```python
from build123d import *

# Parameters (mm, degrees)
F0_R     = 1.75
F0_R_2   = 1
F1_DEPTH = 5.6
F3_W     = 0.9
F3_H     = 5.5
F4_DEPTH = 5.95
F5_R     = 3.5
F5_R_2   = 1.75
F6_DEPTH = 4.2
F7_R     = 2.5
F8_DEPTH = 8


with BuildPart() as f1:
    # F0 (on Front) → F1 (new body)
    with BuildSketch(Plane.XZ):
        with BuildLine():
            Line((-26.9, -2), (-26.9, 0))
            ThreePointArc((-26.9, 0), (-28.8, 1.9), (-30.7, 0))
            Line((-30.7, 0), (-30.7, -2))
            ThreePointArc((-30.7, -2), (-30.1435028843, -3.3435028843), (-28.8, -3.9))
            ThreePointArc((-28.8, -3.9), (-24.6294135718, -5.596855554), (-20.3538194655, -7.0083813116))
            Line((-20.3538194655, -7.0083813116), (-20.7757003916, -8.4478313747))
            ThreePointArc((-20.7757003916, -8.4478313747), (-16.6769659984, -9.5120684601), (-12.5200691265, -10.3198014574))
            Line((-12.5200691265, -10.3198014574), (-12.696252722, -11.4056003986))
            ThreePointArc((-12.696252722, -11.4056003986), (-8.0798243817, -11.9962992417), (-3.4341530829, -12.2757163632))
            ThreePointArc((-3.4341530829, -12.2757163632), (0, -15.1), (3.4341530829, -12.2757163632))
            ThreePointArc((3.4341530829, -12.2757163632), (3.235336932, -10.2648614543), (1.9581459203, -8.699023517))
            ThreePointArc((1.9581459203, -8.699023517), (0, -8.1), (-1.9581459203, -8.699023517))
            ThreePointArc((-1.9581459203, -8.699023517), (-14.9928565077, -7.3200147056), (-27.4941674529, -3.3801454123))
            ThreePointArc((-27.4941674529, -3.3801454123), (-27.0548521783, -2.7513049183), (-26.9, -2))
        make_face()
        with Locations((0, -11.6)):
            Circle(F0_R, mode=Mode.SUBTRACT)
        with Locations((-28.8, 0)):
            Circle(F0_R_2, mode=Mode.SUBTRACT)
        with BuildLine():
            ThreePointArc((27.4941674529, -3.3801454123), (14.9928565077, -7.3200147056), (1.9581459203, -8.699023517))
            ThreePointArc((1.9581459203, -8.699023517), (3.235336932, -10.2648614543), (3.4341530829, -12.2757163632))
            ThreePointArc((3.4341530829, -12.2757163632), (8.0798243817, -11.9962992417), (12.696252722, -11.4056003986))
            Line((12.696252722, -11.4056003986), (12.5200691265, -10.3198014574))
            ThreePointArc((12.5200691265, -10.3198014574), (16.6769659984, -9.5120684601), (20.7757003916, -8.4478313747))
            Line((20.7757003916, -8.4478313747), (20.3538194655, -7.0083813116))
            ThreePointArc((20.3538194655, -7.0083813116), (24.6294135718, -5.596855554), (28.8, -3.9))
            ThreePointArc((28.8, -3.9), (30.1435028843, -3.3435028843), (30.7, -2))
            Line((30.7, -2), (30.7, 0))
            ThreePointArc((30.7, 0), (28.8, 1.9), (26.9, 0))
            Line((26.9, 0), (26.9, -2))
            ThreePointArc((26.9, -2), (27.0548521783, -2.7513049183), (27.4941674529, -3.3801454123))
        make_face()
        with Locations((28.8, 0)):
            Circle(F0_R_2, mode=Mode.SUBTRACT)
    extrude(amount=F1_DEPTH)

    # F3 (on offset) → F4 (join, through all)
    with BuildSketch(Plane.XZ.offset(5.95)):
        Polygon((-18.2045984637, -6.0751883598), (-19.0682685015, -5.8220598041), (-20.1370335143, -9.4686666307), (-19.2733634764, -9.7217951863), align=None)
        Polygon((-10.3615155022, -7.6308153564), (-11.2498964541, -7.4866651419), (-12.0347142888, -12.3234058798), (-11.146333337, -12.4675560944), align=None)
        with Locations((-5.25, -10.45)):
            Rectangle(F3_W, F3_H)
        with Locations((5.25, -10.45)):
            Rectangle(F3_W, F3_H)
        Polygon((11.146333337, -12.4675560944), (12.0347142888, -12.3234058798), (11.2498964541, -7.4866651419), (10.3615155022, -7.6308153564), align=None)
        Polygon((20.1370335143, -9.4686666307), (19.0682685015, -5.8220598041), (18.2045984637, -6.0751883598), (19.2733634764, -9.7217951863), align=None)
    extrude(amount=-F4_DEPTH)

    # F5 (on face) → F6 (join)
    with BuildSketch(Plane.XZ.offset(5.6)):
        with Locations((0, -11.6)):
            Circle(F5_R)
        with Locations((0, -11.6)):
            Circle(F5_R_2, mode=Mode.SUBTRACT)
    extrude(amount=F6_DEPTH)

    # F7 (on face) → F8 (cut)
    with BuildSketch(Plane(origin=(0, 0, 0), x_dir=(-1, 0, 0), z_dir=(0, 1, 0))):
        with Locations((0, -11.6)):
            Circle(F7_R)
    extrude(amount=-F8_DEPTH, mode=Mode.SUBTRACT)


solid = f1.part
```
Input: part model. Units: mm. Frame: model coordinates. A direction names the side the tool comes from. Coordinates: 2 decimals unless noted, no trailing zeros. Write each loop counter-clockwise with the first axis right and the second up, starting at its lowest first coordinate (ties: lowest second). Pieces come first, ordered by that corner, then holes. Notation, with made-up numbers: M 82,43 L 117,43 A15 cw 117,50 Z; hole C 86,86.25 d7. An arc over 180 degrees is marked long. Use one line per item in the form item = value.
Q1. Section D-D (x = -16.5). Return loops of the section in (y, z), plus the area to 3 significant figures.
Answer below:
outline = M -5.6,-9.55 L 0,-9.55 L 0,-6.99 L -5.6,-6.99 Z
area = 14.4 mm²
Q2. Section B-B (y = -8.75). Return loops of the section in (x, z), plus the area to 3 significant figures.
Answer below:
outline = C 0,-11.6 d7; hole C 0,-11.6 d3.5
area = 28.9 mm²
Q3. Draft query along Z for faces 4 (the face through (19.09, -3.68, -9.09)), 5 (the face through (8.325, -2.761, -11.973)), 6 (the face through (28.8, -2.8, 1.9)), 7 (the face through (4, -5.6, -10)). Return one class per face: released by +Z, released by -Z, zero draft, split by the parting line, or undercut.
Answer below:
face_4 = undercut
face_5 = released by -Z
face_6 = released by +Z
face_7 = zero draft
Q4. First-contact query: pin 1 (4 mm diameter, centred on x = -0.5, y = -4, fed in from +Z); pin 2 (4 mm diameter, centred on x = -16.5, z = -10.5, fed in from -Y); pin 3 (4.5 mm diameter, centred on x = -9, z = -10.5, fed in from -Y). Flat tips, straight axial feed; report the tip coordinate or a pass-through.
Answer below:
pin_1 = -8.1
pin_2 = -5.6
pin_3 = -5.95
Q5. Material intervals for probe 1 along X at (y, z) = (-7, -11.5); probe 2 along Z at (x, y) = (0, -8.55); probe 3 along X at (y, z) = (-4, -1.5), sorted ascending. Write a range as from..to.
Answer below:
probe_1 = -3.5..-2.5, 2.5..3.5
probe_2 = -15.1..-13.35, -9.85..-8.1
probe_3 = -30.7..-26.9, 26.9..30.7
Q6. Set-up query: faces 1 (the face through (-26.9, -3, -1)), 2 (the face through (20.57, -2.76, -7.74)), 3 (the face through (12, -3.7, -12.1)). Return all of +Z, -Z, +X, -X, +Y, -Y with unobstructed straight access to the full face (end or side cutting, diameter ignored); none if empty.
Answer below:
face_1 = +Z, +Y, -Y
face_2 = +X, +Y, -Y
face_3 = -Y
Q7. Section A-A (x = 0). Return loops of the section in (y, z), plus the area to 3 significant figures.
Answer below:
outline = M -9.8,-15.1 L 0,-15.1 L 0,-14.1 L -8,-14.1 L -8,-13.35 L -9.8,-13.35 Z; M -9.8,-9.85 L -8,-9.85 L -8,-9.1 L 0,-9.1 L 0,-8.1 L -9.8,-8.1 Z
area = 22.3 mm²
Q8. Section C-C (y = -2.25). Count the separate pieces of the cut face and the enclosed holes in it, plus the area to 3 significant figures.
Answer below:
separate_pieces = 1
enclosed_holes = 3
area = 184 mm²
